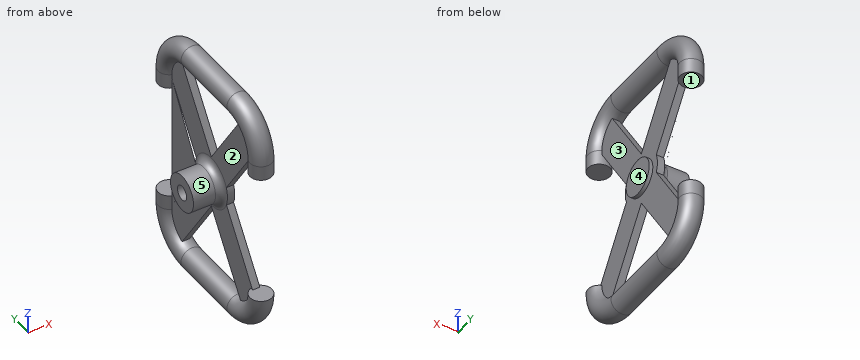
from build123d import *

# Parameters (mm, degrees)
SKETCH14_R          = 1.5
SKETCH15_R          = 1.5
CUT_EXTRUDE4_DEPTH  = 8
SKETCH16_R          = 1
BOSS_EXTRUDE4_DEPTH = 0.5
SKETCH17_R          = 2.5
BOSS_EXTRUDE5_DEPTH = 0.5
SKETCH18_R          = 2.5
SKETCH18_R_2        = 1
BOSS_EXTRUDE6_DEPTH = 4
FILLET2_R           = 1


with BuildPart() as part:
    # Sweep3: sweep along a path in Sketch12
    with BuildLine(Plane(origin=(0, 0, 0), x_dir=(0, 0, -1), z_dir=(1, 0, 0))) as sweep3_path:
        Line((0, 0), (-10, 0))
        ThreePointArc((-10, 0), (-13.535533906, 1.464466094), (-15, 5))
        Line((-15, 5), (-15, 15))
        ThreePointArc((-15, 15), (-13.535533906, 18.535533906), (-10, 20))
        Line((-10, 20), (10, 20))
        ThreePointArc((10, 20), (13.535533906, 18.535533906), (15, 15))
        Line((15, 15), (15, 5))
        ThreePointArc((15, 5), (13.535533906, 1.464466094), (10, 0))
    # Sketch14 → Sweep3 (sweep)
    with BuildSketch(Plane.XY):
        Circle(SKETCH14_R)
    sweep(path=sweep3_path.line)

    # Sketch15 → Cut-Extrude4 (cut, symmetric)
    with BuildSketch(Plane.XY):
        with Locations(Location((0, 0, 0), (0, 0, 270))):
            Circle(SKETCH15_R)
        with Locations((0, 20)):
            Circle(SKETCH15_R)
    extrude(amount=CUT_EXTRUDE4_DEPTH, both=True, mode=Mode.SUBTRACT)


with BuildPart() as cut_extrude4_piece_1:
    # of the separate pieces the step leaves, piece 1, a body of its own (cut_extrude4_pieces)
    add(part.part.solids().sort_by_distance((1.5, 0, 8))[0])



with BuildPart() as cut_extrude4_piece_2:
    # of the separate pieces the step leaves, piece 2, a body of its own (cut_extrude4_pieces)
    add(part.part.solids().sort_by_distance((1.5, 20, -8))[0])


with BuildPart() as cut_extrude4_piece_1_1:
    add(cut_extrude4_piece_1.part)

    add(cut_extrude4_piece_2.part)  # Boss-Extrude4 merges Cut-Extrude4 piece 2
    # Sketch16 → Boss-Extrude4 (add, symmetric)
    with BuildSketch(Plane(origin=(0, 0, 0), x_dir=(0, 0, -1), z_dir=(1, 0, 0))):
        with BuildLine():
            Line((1.301340093, 13.24907894), (11.406580041, 19.892717907))
            ThreePointArc((11.406580041, 19.892717907), (12.616460575, 18.294628285), (13.603996717, 16.550359466))
            Line((13.603996717, 16.550359466), (3.640638612, 10))
            Line((3.640638612, 10), (13.603996717, 3.449640534))
            ThreePointArc((13.603996717, 3.449640534), (12.616460575, 1.705371715), (11.406580041, 0.107282093))
            Line((11.406580041, 0.107282093), (1.301340093, 6.75092106))
            ThreePointArc((1.301340093, 6.75092106), (0, 6.5), (-1.301340093, 6.75092106))
            Line((-1.301340093, 6.75092106), (-11.406580041, 0.107282093))
            ThreePointArc((-11.406580041, 0.107282093), (-12.616460575, 1.705371715), (-13.603996717, 3.449640534))
            Line((-13.603996717, 3.449640534), (-3.640638612, 10))
            Line((-3.640638612, 10), (-13.603996717, 16.550359466))
            ThreePointArc((-13.603996717, 16.550359466), (-12.616460575, 18.294628285), (-11.406580041, 19.892717907))
            Line((-11.406580041, 19.892717907), (-1.301340093, 13.24907894))
            ThreePointArc((-1.301340093, 13.24907894), (0, 13.5), (1.301340093, 13.24907894))
        make_face()
        with Locations((0, 10)):
            Circle(SKETCH16_R, mode=Mode.SUBTRACT)
    extrude(amount=BOSS_EXTRUDE4_DEPTH, both=True)

    # Sketch17 → Boss-Extrude5 (add)
    with BuildSketch(Plane(origin=(0.5, 0, 0), x_dir=(0, 0, -1), z_dir=(1, 0, 0))):
        with Locations((0, 10)):
            Circle(SKETCH17_R)
    extrude(amount=BOSS_EXTRUDE5_DEPTH)

    # Sketch18 → Boss-Extrude6 (add)
    with BuildSketch(Plane.ZY.offset(0.5)):
        with Locations(Location((0, 10, 0), (0, 0, 180))):
            Circle(SKETCH18_R)
        with Locations((0, 10)):
            Circle(SKETCH18_R_2, mode=Mode.SUBTRACT)
    extrude(amount=BOSS_EXTRUDE6_DEPTH)

    # Fillet2
    fillet2_edges = [cut_extrude4_piece_1_1.edges().sort_by_distance(p)[0] for p in [
        (-0.5, 10, 2.5),
    ]]
    fillet(fillet2_edges, radius=FILLET2_R - 0.0001)  # a hair under: the kernel refuses the full size


solid = cut_extrude4_piece_1_1.part
Can you work these out from the model? Positions are in its coordinate system, mm. Face numbers are marked on the shaded views. A direction names the side the tool comes from. Coordinates: 2 decimals unless noted, no trailing zeros. Order: outer loops, then holes, each group sorted by start corner. A loop starts at its lowest first (then second) coordinate and runs counter-clockwise, first axis right, second up. Notation, with made-up numbers: M 4,24 L 38,24 A28 ccw 38,46 Z; hole C 41,25 d1. An arc over 180 degrees is marked long. Write item = value, one per line.
(1) For pin 1 Ø1.5 at (x, y) = (-0.5, 0) entering from -Z; pin 2 Ø3 at (y, z) = (10.5, 13) entering from -X; pin 3 Ø0.9 at (x, y) = (0, -0.5) entering from +Z; pin 4 Ø9 at (y, z) = (13.5, -6) entering from -X, each with a flat end and sliding along its axis, tell me the tip position at first contact or that it passes through.
Results are:
pin_1 = -14.85
pin_2 = -1.41
pin_3 = 14.09
pin_4 = -4.5
(2) Suppose I cut it at C-C on y = 6. Please give me the cut outline in (x, z), plus the area to 3 significant figures.
Results are:
outline = C 0,-15 d3; C 0,15 d3; M -0.5,-9.72 L 0.5,-9.72 L 0.5,-2.44 L -0.5,-2.44 Z; M -0.5,2.44 L 0.5,2.44 L 0.5,9.72 L -0.5,9.72 Z
area = 28.7 mm2
(3) Suppose I cut it at D-D on z = -9. Please give me the cut outline in (x, y), plus the area to 3 significant figures.
Results are:
outline = C 0,20 d3; M -0.5,1.69 L 0.5,1.69 L 0.5,6.48 L -0.5,6.48 Z; M -0.5,13.52 L 0.5,13.52 L 0.5,18.31 L -0.5,18.31 Z
area = 16.6 mm2
(4) For the marked faces 1, 2 and 3, which set-ups out of +Z, -Z, +X, -X, +Y, -Y let a thin tool reach every point of the face, with its end or its side?
Results are:
face_1 = +X, -X, +Y
face_2 = -X
face_3 = +X
(5) Suppose I cut it at A-A on z = 6. Please give me the cut outline in (x, y).
Results are:
outline = M -0.5,3.66 L 0.5,3.66 L 0.5,8.45 L -0.5,8.45 Z; M -0.5,11.55 L 0.5,11.55 L 0.5,16.34 L -0.5,16.34 Z
(6) If we mould it in two halves opening along Z, with no side actions, what happens to the marked faces 4 and 5? For each: pulls with the +Z half, pulls with the -Z half, needs draft (parallel to the pull), parting line crosses it, or undercut.
Results are:
face_4 = undercut
face_5 = parting line crosses it
(7) I need wall thicknesses on line 1 along Y through (x, z) = (-3.65, 0); line 2 along Z through (x, y) = (-3.7, 10); line 3 along X through (y, z) = (17, 9). Which ranges of each line are inside material? Lowest first, please. Write a range as [from, to].
Results are:
line_1 = [7.5, 9], [11, 12.5]
line_2 = [-2.5, -1], [1, 2.5]
line_3 = [-0.5, 0.5]
